```python
from build123d import *

# Parameters (mm, degrees)
SKETCH18_W              = 228.04
SKETCH18_H              = 171.92
BOSS_EXTRUDE6_DEPTH     = 26.5
SKETCH20_W              = 218.04
SKETCH20_H              = 171.92
CUT_EXTRUDE6_DEPTH      = 21.5
SKETCH22_W              = 228.04
SKETCH22_H              = 18.7
BOSS_EXTRUDE7_DEPTH     = 26.5
SKETCH23_W              = 228.04
SKETCH23_H              = 18.7
BOSS_EXTRUDE8_DEPTH     = 26.5
SKETCH24_W              = 175
SKETCH24_H              = 18.7
CUT_EXTRUDE7_DEPTH      = 3.35
SKETCH25_W              = 175
SKETCH25_H              = 18.7
CUT_EXTRUDE8_DEPTH      = 3.35
SKETCH27_W              = 175
SKETCH27_H              = 12.7
CUT_EXTRUDE9_DEPTH      = 3
SKETCH28_W              = 175
SKETCH28_H              = 12.7
CUT_EXTRUDE10_DEPTH     = 3
SKETCH31_R              = 1.65
SKETCH31_R_2            = 1.651
CUT_EXTRUDE15_DEPTH     = 1.825
CUT_EXTRUDE17_DEPTH     = 3.175
SKETCH39_R              = 2.2
CUT_EXTRUDE18_DEPTH     = 26.5
SKETCH40_R              = 4.4
CUT_EXTRUDE19_DEPTH     = 20.9
FILLET1_R               = 3.81
CUT_EXTRUDE20_DEPTH     = 3.6
SKETCH47_R              = 3.3782
BOSS_EXTRUDE14_DEPTH    = 10.16
MIRROR8_COPY_1_SKETCH_R = 2.2
MIRROR8_COPY_1_DEPTH    = 26.5
MIRROR8_COPY_2_SKETCH_R = 4.4
MIRROR8_COPY_2_DEPTH    = 20.9
MIRROR8_COPY_3_DEPTH    = 3.6


with BuildPart() as part:
    # Sketch18 → Boss-Extrude6 (new body)
    with BuildSketch(Plane(origin=(0, 0, 0), x_dir=(1, 0, 0), z_dir=(0, 1, 0))):
        Rectangle(SKETCH18_W, SKETCH18_H)
    extrude(amount=BOSS_EXTRUDE6_DEPTH)

    # Sketch20 → Cut-Extrude6 (cut)
    with BuildSketch(Plane(origin=(0, 26.5, 0), x_dir=(1, 0, 0), z_dir=(0, 1, 0))):
        Rectangle(SKETCH20_W, SKETCH20_H)
    extrude(amount=-CUT_EXTRUDE6_DEPTH, mode=Mode.SUBTRACT)

    # Sketch22 → Boss-Extrude7 (add)
    with BuildSketch(Plane(origin=(0, 0, 0), x_dir=(1, 0, 0), z_dir=(0, 1, 0))):
        with Locations((0, -95.31)):
            Rectangle(SKETCH22_W, SKETCH22_H)
    extrude(amount=BOSS_EXTRUDE7_DEPTH)

    # Sketch23 → Boss-Extrude8 (add)
    with BuildSketch(Plane(origin=(0, 0, 0), x_dir=(1, 0, 0), z_dir=(0, 1, 0))):
        with Locations((0, 95.31)):
            Rectangle(SKETCH23_W, SKETCH23_H)
    extrude(amount=BOSS_EXTRUDE8_DEPTH)

    # Sketch24 → Cut-Extrude7 (cut)
    with BuildSketch(Plane(origin=(0, 26.5, 0), x_dir=(1, 0, 0), z_dir=(0, 1, 0))):
        with Locations((0, 95.31)):
            Rectangle(SKETCH24_W, SKETCH24_H)
    extrude(amount=-CUT_EXTRUDE7_DEPTH, mode=Mode.SUBTRACT)

    # Sketch25 → Cut-Extrude8 (cut)
    with BuildSketch(Plane(origin=(0, 26.5, 0), x_dir=(1, 0, 0), z_dir=(0, 1, 0))):
        with Locations((0, -95.31)):
            Rectangle(SKETCH25_W, SKETCH25_H)
    extrude(amount=-CUT_EXTRUDE8_DEPTH, mode=Mode.SUBTRACT)

    # Sketch27 → Cut-Extrude9 (cut)
    with BuildSketch(Plane(origin=(0, 23.15, 0), x_dir=(1, 0, 0), z_dir=(0, 1, 0))):
        with Locations((0, -95.31)):
            Rectangle(SKETCH27_W, SKETCH27_H)
    extrude(amount=-CUT_EXTRUDE9_DEPTH, mode=Mode.SUBTRACT)

    # Sketch28 → Cut-Extrude10 (cut)
    with BuildSketch(Plane(origin=(0, 23.15, 0), x_dir=(1, 0, 0), z_dir=(0, 1, 0))):
        with Locations((0, 95.31)):
            Rectangle(SKETCH28_W, SKETCH28_H)
    extrude(amount=-CUT_EXTRUDE10_DEPTH, mode=Mode.SUBTRACT)

    # Sketch31 → Cut-Extrude15 (cut)
    with BuildSketch(Plane(origin=(0, 5, 0), x_dir=(1, 0, 0), z_dir=(0, 1, 0))):
        with Locations(Location((-82.448, 57.15, 0), (0, 0, 270))):
            Circle(SKETCH31_R)
        with Locations(Location((101.448, 57.15, 0), (0, 0, 270))):
            Circle(SKETCH31_R_2)
        with Locations(Location((101.448, -57.15, 0), (0, 0, 270))):
            Circle(SKETCH31_R_2)
        with Locations(Location((-82.448, -57.15, 0), (0, 0, 270))):
            Circle(SKETCH31_R)
    extrude(amount=-CUT_EXTRUDE15_DEPTH, mode=Mode.SUBTRACT)

    # Sketch33 → Cut-Extrude17 (cut)
    with BuildSketch(Plane.XZ):
        Polygon((-79.316971755, -58.9577), (-79.316971755, -55.3423), (-82.448, -53.5346), (-85.579028245, -55.3423), (-85.579028245, -58.9577), (-82.448, -60.7654), align=None)
        Polygon((104.579028245, -58.9577), (104.579028245, -55.3423), (101.448, -53.5346), (98.316971755, -55.3423), (98.316971755, -58.9577), (101.448, -60.7654), align=None)
        Polygon((-79.316971755, 58.9577), (-82.448, 60.7654), (-85.579028245, 58.9577), (-85.579028245, 55.3423), (-82.448, 53.5346), (-79.316971755, 55.3423), align=None)
        Polygon((98.316971755, 58.9577), (98.316971755, 55.3423), (101.448, 53.5346), (104.579028245, 55.3423), (104.579028245, 58.9577), (101.448, 60.7654), align=None)
    extrude(amount=-CUT_EXTRUDE17_DEPTH, mode=Mode.SUBTRACT)

    # Sketch39 → Cut-Extrude18 (cut)
    with BuildSketch(Plane(origin=(0, 26.5, 0), x_dir=(1, 0, 0), z_dir=(0, 1, 0))):
        with Locations(Location((100.76, 95.31, 0), (0, 0, 270))):
            Circle(SKETCH39_R)
    cut_extrude18 = extrude(amount=-CUT_EXTRUDE18_DEPTH, mode=Mode.SUBTRACT)

    # Sketch40 → Cut-Extrude19 (cut)
    with BuildSketch(Plane.XZ):
        with Locations(Location((100.76, -95.31, 0), (0, 0, 270))):
            Circle(SKETCH40_R)
    cut_extrude19 = extrude(amount=-CUT_EXTRUDE19_DEPTH, mode=Mode.SUBTRACT)

    # Mirror3: Cut-Extrude18 across plane
    add(cut_extrude18.mirror(Plane.XY), mode=Mode.SUBTRACT)

    # Mirror4: Cut-Extrude19 across plane
    add(cut_extrude19.mirror(Plane.XY), mode=Mode.SUBTRACT)

    # Fillet1
    fillet1_edges = [part.edges().sort_by_distance(p)[0] for p in [
        (-114.02, 13.25, 104.66),
        (114.02, 13.25, 104.66),
        (114.02, 13.25, -104.66),
        (-114.02, 13.25, -104.66),
    ]]
    fillet(fillet1_edges, radius=FILLET1_R)

    # Sketch41 → Cut-Extrude20 (cut)
    with BuildSketch(Plane(origin=(0, 26.5, 0), x_dir=(1, 0, 0), z_dir=(0, 1, 0))):
        Polygon((98.681539031, -91.71), (96.603078062, -95.31), (98.681539031, -98.91), (102.838460969, -98.91), (104.916921938, -95.31), (102.838460969, -91.71), align=None)
    cut_extrude20 = extrude(amount=-CUT_EXTRUDE20_DEPTH, mode=Mode.SUBTRACT)

    # Mirror5: Cut-Extrude20 across plane
    add(cut_extrude20.mirror(Plane.XY), mode=Mode.SUBTRACT)

    # Sketch47 → Boss-Extrude14 (add)
    # profile 1 of 2: a face of its own
    with BuildSketch(Plane.XZ):
        with BuildLine():
            ThreePointArc((-48.903154853, -113.757225166), (-47.210651626, -109.12978233), (-45.13728714, -104.66))
            Line((-45.13728714, -104.66), (-57.122870876, -104.66))
            Line((-57.122870876, -104.66), (-68.88271286, -104.66))
            ThreePointArc((-68.88271286, -104.66), (-66.809348374, -109.12978233), (-65.116845147, -113.757225166))
            ThreePointArc((-65.116845147, -113.757225166), (-57.01, -120.350559583), (-48.903154853, -113.757225166))
        make_face()
        with Locations(Location((-57.01, -112.07, 0), (0, 0, 270))):
            Circle(SKETCH47_R, mode=Mode.SUBTRACT)
    # profile 2 of 2: a face of its own
    with BuildSketch(Plane.XZ):
        with BuildLine():
            ThreePointArc((45.13728714, -104.66), (47.210651626, -109.12978233), (48.903154853, -113.757225166))
            ThreePointArc((48.903154853, -113.757225166), (57.01, -120.350559583), (65.116845147, -113.757225166))
            ThreePointArc((65.116845147, -113.757225166), (66.809348374, -109.12978233), (68.88271286, -104.66))
            Line((68.88271286, -104.66), (57.122870876, -104.66))
            Line((57.122870876, -104.66), (45.13728714, -104.66))
        make_face()
        with Locations(Location((57.01, -112.07, 0), (0, 0, 270))):
            Circle(SKETCH47_R, mode=Mode.SUBTRACT)
    boss_extrude14 = extrude(amount=-BOSS_EXTRUDE14_DEPTH)

    # Mirror6: Boss-Extrude14 across plane
    add(boss_extrude14.mirror(Plane.XY))

    # Mirror8: Cut-Extrude18, Cut-Extrude19, Cut-Extrude20 across plane
    add(cut_extrude18.mirror(Plane.ZY.offset(-0.02)), mode=Mode.SUBTRACT)
    add(cut_extrude19.mirror(Plane.ZY.offset(-0.02)), mode=Mode.SUBTRACT)
    add(cut_extrude20.mirror(Plane.ZY.offset(-0.02)), mode=Mode.SUBTRACT)

    # Mirror8 copy 1 sketch → Mirror8 copy 1 (cut)
    with BuildSketch(Plane(origin=(0.04, 26.5, 0), x_dir=(-1, 0, 0), z_dir=(0, 1, 0))):
        with Locations(Location((100.76, 95.31, 0), (0, 0, 270))):
            Circle(MIRROR8_COPY_1_SKETCH_R)
    extrude(amount=-MIRROR8_COPY_1_DEPTH, mode=Mode.SUBTRACT)

    # Mirror8 copy 2 sketch → Mirror8 copy 2 (cut)
    with BuildSketch(Plane(origin=(0.04, 0, 0), x_dir=(-1, 0, 0), z_dir=(0, -1, 0))):
        with Locations(Location((100.76, -95.31, 0), (0, 0, 270))):
            Circle(MIRROR8_COPY_2_SKETCH_R)
    extrude(amount=-MIRROR8_COPY_2_DEPTH, mode=Mode.SUBTRACT)

    # Mirror8 copy 3 sketch → Mirror8 copy 3 (cut)
    with BuildSketch(Plane(origin=(0.04, 26.5, 0), x_dir=(-1, 0, 0), z_dir=(0, 1, 0))):
        Polygon((98.681539031, -91.71), (96.603078062, -95.31), (98.681539031, -98.91), (102.838460969, -98.91), (104.916921938, -95.31), (102.838460969, -91.71), align=None)
    extrude(amount=-MIRROR8_COPY_3_DEPTH, mode=Mode.SUBTRACT)


solid = part.part
```
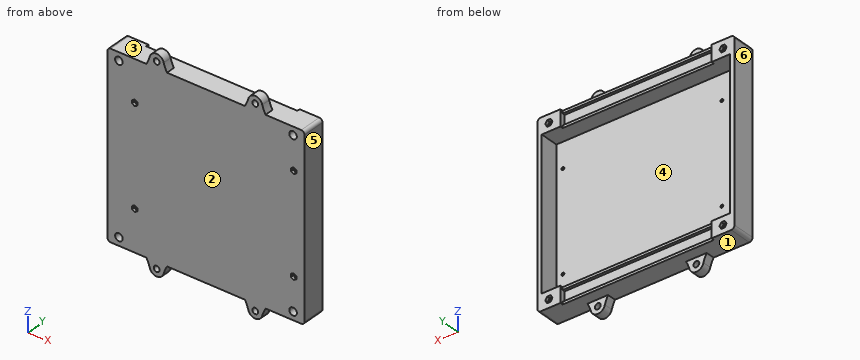
CAD build for the part. Positions are in the model's coordinates, mm. Face numbers are marked on the shaded views. A direction names the side the tool comes from. Coordinates: 2 decimals unless noted, no trailing zeros. Order: outer loops, then holes, each group sorted by start corner. A loop starts at its lowest first (then second) coordinate and runs counter-clockwise, first axis right, second up. Notation, with made-up numbers: M 29,-12 L 78,-12 A22 cw 78,23 Z; hole C 56.5,15 d5. An arc over 180 degrees is marked long. Write each question's results on one line, items separated by ' | '. Start each with the question number.
Q1. Drill centre lines: probe 1 along X at (y, z) = (21.65, -95.31); probe 2 along Z at (x, y) = (55, 22.25); probe 3 along X at (y, z) = (4.2, -57.15). Where is each one in solid material? Low to high. Write a range as from..to.
Q2. Cut at B-B (x = -26). List the corners of the cut face in (y, z), then the cut area to 3 significant figures.
Q3. Pull direction X, two halves, no side cores. Call the marked faces 3, 4, 5 and 6: +X half, -X half, draft (parallel to the pull), parting line (faces both ways), or undercut.
Q4. Flat gauge pins, fed straight in: P1, Ø17.5, axis at x = -54.5, z = -113.5, coming from the +Y side; P2, Ø1.5, axis at x = 88.5, y = 11.5, coming from the -Z side; P3, Ø4, axis at x = -22.5, z = 73, coming from the +Y side. Where does each tip first touch, or does it go through?
Q5. Which spindle directions (+Z, -Z, +X, -X, +Y, -Y) get a long thin tool onto all of the face, cutting with end or side? Do the marked faces 1 and 2. Say none if no direction does.
Q6. Cut at A-A (z = 41.5). List the corners of the cut face in (x, y).
Found:
1) probe 1: -114.02..-102.92, -98.52..-87.5, 87.5..98.56, 102.96..114.02 | probe 2: -104.66..-101.66, -88.96..-85.96, 85.96..88.96, 101.66..104.66 | probe 3: -114.02..-84.1, -80.8..99.8, 103.1..114.02
2) outline: M 0,-104.66 L 23.15,-104.66 L 23.15,-101.66 L 20.15,-101.66 L 20.15,-88.96 L 23.15,-88.96 L 23.15,-85.96 L 5,-85.96 L 5,85.96 L 23.15,85.96 L 23.15,88.96 L 20.15,88.96 L 20.15,101.66 L 23.15,101.66 L 23.15,104.66 L 0,104.66 Z | area: 1,650 mm²
3) face 3: undercut | face 4: undercut | face 5: +X half | face 6: -X half
4) P1: y = 10.16 | P2: z = -104.66 | P3: y = 5
5) face 1: -Z, +Y | face 2: +Z, -Z, +X, -X, -Y
6) outline: M -114.02,0 L 114.02,0 L 114.02,26.5 L 109.02,26.5 L 109.02,5 L -109.02,5 L -109.02,26.5 L -114.02,26.5 Z
